from build123d import *

# Parameters (mm, degrees)
F0_W     = 2819.4
F0_H     = 762
F1_DEPTH = 304.8
F2_W     = 838.2
F2_H     = 381
F3_DEPTH = 304.8
F4_W     = 304.8
F4_H     = 838.2
F5_DEPTH = 76.2


with BuildPart() as f1:
    # F0 (on Right) → F1 (new body)
    with BuildSketch(Plane.YZ):
        Rectangle(F0_W, F0_H)
    extrude(amount=F1_DEPTH)

    # F2 (on face) → F3 (cut)
    with BuildSketch(Plane.YZ.offset(304.8)):
        with Locations((-76.2, -190.5)):
            Rectangle(F2_W, F2_H)
    extrude(amount=-F3_DEPTH, mode=Mode.SUBTRACT)

    # F4 (on face) → F5 (join)
    with BuildSketch(Plane.XY.offset(381)):
        with Locations((152.4, -76.2)):
            Rectangle(F4_W, F4_H)
    extrude(amount=F5_DEPTH)


solid = f1.part
Source: CAD feature listing. Evaluate the final solid. Frame: model axes, mm. A direction names the side the tool comes from. Round coordinates to 2 decimals unless told otherwise and drop trailing zeros. Write each loop counter-clockwise with the first axis right and the second up, starting at its lowest first coordinate (ties: lowest second). Pieces come first, ordered by that corner, then holes. Notation, with made-up numbers: M 7,-4.5 L 62,-4.5 A8 ccw 62,9.5 Z; hole C -4,65 d11. An arc over 180 degrees is marked long. One line per item, written item: value. Start each with the question number.
Item 1: Ray query, L1, parallel to Y at x = 29, z = -4; L2, parallel to Y at x = 160.5, z = 412; L3, parallel to Z at x = 253, y = -62.5. Return the intervals inside material, ascending. Write a range as from..to.
Item 2: Mould query, pull axis Y, two halves, no side actions, for faces 5 (the flat face through (150, 869, 381)), 6 (the flat face through (150, 1409.7, -5)), 7 (the flat face through (155, -495.3, -193)), 8 (the flat face through (155, -82, 0)). Classes: pulls with the +Y half, pulls with the -Y half, needs draft (parallel to the pull), parting line crosses it, or undercut.
Item 3: Section query A-A (z = -262). Return the cut outline in (x, y), plus the area to 3 significant figures.
Item 4: Set-up query: faces 1 (the flat face through (150, -495.3, 419)), 2 (the flat face through (155, 342.9, -193)), 3 (the flat face through (150, 869, -381)), 4 (the flat face through (150, 342.9, 419)). Return all of +Z, -Z, +X, -X, +Y, -Y with unobstructed straight access to the full face (end or side cutting, diameter ignored); none if empty.
Item 5: Pin query (flat end, axial travel): pin 1 (8 mm diameter, centred on x = 232, y = 86.5, fed in from -Z); pin 2 (6 mm diameter, centred on x = 199.5, y = 941, fed in from +Z). Return the tip coordinate at first contact, or that it passes through.
Item 6: Section query D-D (y = 286.5). Return the cut outline in (x, z), plus the area to 3 significant figures.
Item 7: Section query B-B (x = 62). Return the cut outline in (y, z), plus the area to 3 significant figures.
Item 8: Section query C-C (y = -804). Return the cut outline in (x, z).
Result set:
1. L1: y = -1409.7..-495.3, 342.9..1409.7
1. L2: y = -495.3..342.9
1. L3: z = 0..457.2
2. face 5: needs draft
2. face 6: pulls with the +Y half
2. face 7: undercut
2. face 8: undercut
3. outline: M 0,-1409.7 L 304.8,-1409.7 L 304.8,-495.3 L 0,-495.3 Z; M 0,342.9 L 304.8,342.9 L 304.8,1409.7 L 0,1409.7 Z
3. area: 604,000 mm²
4. face 1: +Z, +X, -X, -Y
4. face 2: -Z, +X, -X
4. face 3: -Z, +X, -X, +Y, -Y
4. face 4: +Z, +X, -X, +Y
5. pin 1: stops at z = 0
5. pin 2: stops at z = 381
6. outline: M 0,0 L 304.8,0 L 304.8,457.2 L 0,457.2 Z
6. area: 139,000 mm²
7. outline: M -1409.7,-381 L -495.3,-381 L -495.3,0 L 342.9,0 L 342.9,-381 L 1409.7,-381 L 1409.7,381 L 342.9,381 L 342.9,457.2 L -495.3,457.2 L -495.3,381 L -1409.7,381 Z
7. area: 1,890,000 mm²
8. outline: M 0,-381 L 304.8,-381 L 304.8,381 L 0,381 Z
